from build123d import *

# Parameters (mm, degrees)
BOSS_EXTRUDE1_DEPTH = 3
SKETCH2_R           = 4
CUT_EXTRUDE1_DEPTH  = 13
SKETCH3_R           = 1
CUT_EXTRUDE2_DEPTH  = 13
SKETCH4_R           = 1
CUT_EXTRUDE3_DEPTH  = 3


with BuildPart() as part:
    # Sketch1 → Boss-Extrude1 (new body)
    with BuildSketch(Plane(origin=(0, 0, 0), x_dir=(1, 0, 0), z_dir=(0, 1, 0))):
        with BuildLine():
            Line((-10, 0), (-14, -25))
            Line((-14, -25), (14, -25))
            Line((14, -25), (10, 0))
            ThreePointArc((10, 0), (0, 10), (-10, 0))
        make_face()
    extrude(amount=BOSS_EXTRUDE1_DEPTH)

    # Sketch2 → Cut-Extrude1 (cut)
    with BuildSketch(Plane(origin=(0, 3, 0), x_dir=(1, 0, 0), z_dir=(0, 1, 0))):
        Circle(SKETCH2_R)
    extrude(amount=-CUT_EXTRUDE1_DEPTH, mode=Mode.SUBTRACT)

    # Sketch3 → Cut-Extrude2 (cut)
    with BuildSketch(Plane(origin=(0, 3, 0), x_dir=(1, 0, 0), z_dir=(0, 1, 0))):
        with Locations((-6.52, -19)):
            Circle(SKETCH3_R)
        with Locations((6.52, -19)):
            Circle(SKETCH3_R)
        with Locations((0, -19)):
            Circle(SKETCH3_R)
    extrude(amount=-CUT_EXTRUDE2_DEPTH, mode=Mode.SUBTRACT)

    # Sketch4 → Cut-Extrude3 (cut)
    with BuildSketch(Plane(origin=(0, 3, 0), x_dir=(1, 0, 0), z_dir=(0, 1, 0))):
        with Locations((0, -7)):
            Circle(SKETCH4_R)
        with Locations((-7, 0)):
            Circle(SKETCH4_R)
        with Locations((0, 7)):
            Circle(SKETCH4_R)
        with Locations((7, 0)):
            Circle(SKETCH4_R)
    extrude(amount=-CUT_EXTRUDE3_DEPTH, mode=Mode.SUBTRACT)


solid = part.part
Model file for the job. Use its own axes, mm. Give positions to 0.01 mm unless a question says otherwise; leave off trailing zeros. Write each loop counter-clockwise with the first axis right and the second up, starting at its lowest first coordinate (ties: lowest second). Pieces come first, ordered by that corner, then holes. Notation, with made-up numbers: M 2.25,13.5 L 44.25,13.5 A34 ccw 44.25,43.5 Z; hole C 31.5,-21 d10. An arc over 180 degrees is marked long. One line per item, written item: value. Start each with the question number.
Q1. Saw through at B-B, the plane x = -7. Write the cut outline in (y, z).
Q2. Saw through at A-A, the plane x = 0. Write the cut outline in (y, z), plus the area to 3 significant figures.
Q3. Drop a flat-ended pin along its axis: pin 1 Ø1.5 at (x, y) = (-4, 1.5) entering from -Z. Give the stop position or say it passes through.
Q4. Two-plate mould, pull along Z, no slides. Class faces 1 (the flat face through (12.028, 1.479, 12.675)), 2 (the flat face through (0, 0, 11)), 3 (the cylindrical face through (6.2, 1.5, 0.6)), 4 (the flat face through (0, 1, 25)): +Z half, -Z half, draft (parallel to the pull), parting line (faces both ways), or undercut.
Q5. Saw through at C-C, the plane z = 19.5. Write the cut outline in (x, y).
Q6. Saw through at D-D, the plane z = 10. Write the cut outline in (x, y), plus the area to 3 significant figures.
Q7. Probe probe 1 along X at (y, z) = (0.9, 0); probe 2 along Z at (x, y) = (0, 1.45); probe 3 along X at (y, z) = (0.95, 19). List the from-to ranges inside material, lowest first. Write a range as [from, to].
Output values:
1. outline: M 0,-7.14 L 3,-7.14 L 3,-1 L 0,-1 Z; M 0,1 L 3,1 L 3,18.12 L 0,18.12 Z; M 0,19.88 L 3,19.88 L 3,25 L 0,25 Z
2. outline: M 0,-10 L 3,-10 L 3,-8 L 0,-8 Z; M 0,-6 L 3,-6 L 3,-4 L 0,-4 Z; M 0,4 L 3,4 L 3,6 L 0,6 Z; M 0,8 L 3,8 L 3,18 L 0,18 Z; M 0,20 L 3,20 L 3,25 L 0,25 Z
2. area: 63.0 mm²
3. pin 1: stops at z = -9.46
4. face 1: -Z half
4. face 2: draft
4. face 3: undercut
4. face 4: +Z half
5. outline: M -13.12,0 L -7.39,0 L -7.39,3 L -13.12,3 Z; M -5.65,0 L -0.87,0 L -0.87,3 L -5.65,3 Z; M 0.87,0 L 5.65,0 L 5.65,3 L 0.87,3 Z; M 7.39,0 L 13.12,0 L 13.12,3 L 7.39,3 Z
6. outline: M -11.6,0 L 11.6,0 L 11.6,3 L -11.6,3 Z
6. area: 69.6 mm²
7. probe 1: x = [-10, -8], [-6, -4], [4, 6], [8, 10]
7. probe 2: z = [-10, -8], [-6, -4], [4, 6], [8, 18], [20, 25]
7. probe 3: x = [-13.04, -7.52], [-5.52, -1], [1, 5.52], [7.52, 13.04]
